Geometry: see drawing. Coordinates: mm, zero at the bounding-box minimum. Give positions to 0.01 mm unless a question says otherwise; leave off trailing zeros. Order: outer loops, then holes, each group sorted by start corner. A loop starts at its lowest first (then second) coordinate and runs counter-clockwise, first axis right, second up. Notation, with made-up numbers: M -14.75,-14 L 3.25,-14 A25 ccw 3.25,16 Z; hole C 27.25,30.25 d4. An arc over 180 degrees is marked long. Use a Markdown table: item, result.
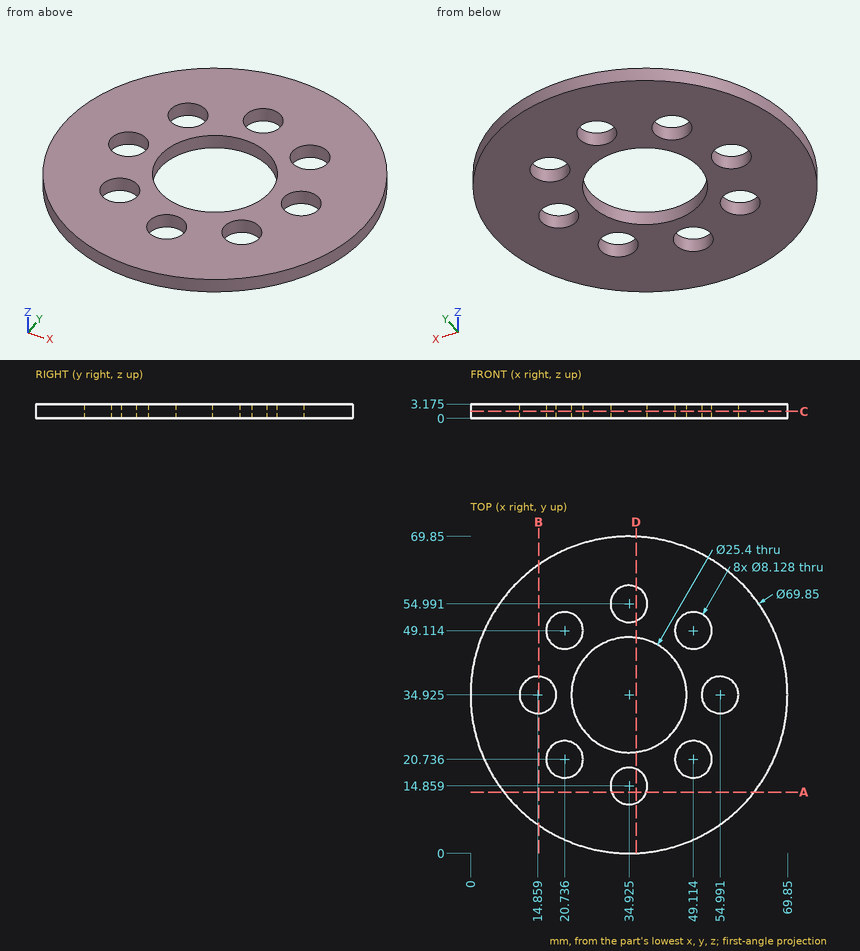
1) Cut plane B-B on x = 15. Return loops of the section in (y, z) (1 decimal).
Response values:
| item | result |
|---|---|
| outline | M 6.2,0 L 30.9,0 L 30.9,3.2 L 6.2,3.2 Z; M 39,0 L 63.6,0 L 63.6,3.2 L 39,3.2 Z |
2) Cut plane C-C on z = 1.55. State how many separate pieces and enclosed holes the cut face has, and give its area (3 significant figures).
Response values:
| item | result |
|---|---|
| separate pieces | 1 |
| enclosed holes | 9 |
| area | 2,910 mm² |
3) First-contact query: pin 1 Ø1.5 at (x, z) = (41, 2.5) entering from +Y; pin 2 Ø6.5 at (x, y) = (49.11, 49.11) entering from +Z; pin 3 Ø1.5 at (y, z) = (36.5, 1) entering from +X; pin 4 Ø1.5 at (x, z) = (48, 2) entering from -Y. Flat tips, straight axial feed; report the tip coordinate or a pass-through.
Response values:
| item | result |
|---|---|
| pin 1 | stops at y = 69.44 |
| pin 2 | passes through |
| pin 3 | stops at x = 69.84 |
| pin 4 | stops at y = 2.25 |
4) Cut plane D-D on x = 36.5. Return loops of the section in (y, z) (1 decimal).
Response values:
| item | result |
|---|---|
| outline | M 0,0 L 11.1,0 L 11.1,3.2 L 0,3.2 Z; M 18.6,0 L 22.3,0 L 22.3,3.2 L 18.6,3.2 Z; M 47.5,0 L 51.2,0 L 51.2,3.2 L 47.5,3.2 Z; M 58.7,0 L 69.8,0 L 69.8,3.2 L 58.7,3.2 Z |
5) Material intervals for line 1 (Y direction, x = 32.5, z = 1.1) (1 decimal); line 2 (Y direction, x = 46, z = 0.2) (1 decimal); line 3 (X direction, y = 44.5, z = 1.65), sorted ascending. Write a range as from..to.
Response values:
| item | result |
|---|---|
| line 1 | y = 0.1..11.6, 18.1..22.5, 47.4..51.7, 58.3..69.8 |
| line 2 | y = 1.8..18.1, 23.3..28.7, 41.1..46.5, 51.7..68 |
| line 3 | x = 1.34..26.58, 43.27..68.51 |
6) Cut plane A-A on y = 13.5. Return loops of the section in (x, z) (1 decimal).
Response values:
| item | result |
|---|---|
| outline | M 7.3,0 L 31.1,0 L 31.1,3.2 L 7.3,3.2 Z; M 38.8,0 L 62.5,0 L 62.5,3.2 L 38.8,3.2 Z |
